Here's how the part is built. I have some questions about the finished solid (model axes, mm). A direction names the side the tool comes from. Coordinates: 2 decimals unless noted, no trailing zeros. Order: outer loops, then holes, each group sorted by start corner. A loop starts at its lowest first (then second) coordinate and runs counter-clockwise, first axis right, second up. Notation, with made-up numbers: (-9, 43.5) - (8, 43.5) arc R17 cw to (8, 69.5) - close; hole circle Ø8 at (-25.5, 50). An arc over 180 degrees is marked (long way). Answer in a Markdown table with one row per item. Add a question column.
Item 1: Will these pins go through, and if not, where does the flat tip stop? pin 1 Ø1 at (y, z) = (-5.5, -0.5) entering from +X; pin 2 Ø1.6 at (x, z) = (3, -0.5) entering from -Y; pin 3 Ø1 at (y, z) = (-7, 0.5) entering from -X.
Item 2: If I drill on line 1 along X through (y, z) = (-5, 1.4); line 2 along Y through (x, z) = (-10.5, -0.35), over which ranges is the centre line in solid material (lowest first)? Write a range as from..to.
Item 3: I want a section at C-C (x = 5). Please give me the cut outline in (y, z), plus the area to 3 significant figures.
Item 4: I want a section at A-A (y = -6). Please give me the cut outline in (x, z).
Item 5: I want a section at B-B (z = 0). Please give me the cut outline in (x, y).
Item 6: On a 3-axis mill with a long thin cutter (end or side, diameter ignored), from which of +Z, -Z, +X, -X, +Y, -Y can I reach the whole of each face in a straight line? I mean faces 1 (the flat face through (-38.202, -6, 0)), 2 (the flat face through (0, -4.864, 0)), 3 (the flat face through (40, -4.864, 0)). Say none if no direction works.
```python
from build123d import *

# Parameters (mm, degrees)
BOSS_EXTRUDE1_DEPTH = 1.5875
BOSS_EXTRUDE2_DEPTH = 3.175


with BuildPart() as part:
    # Sketch1 → Boss-Extrude1 (new body, symmetric)
    with BuildSketch(Plane.XY):
        Polygon((-12.6492, -4.7625), (12.7, -4.7625), (12.7, -7.9375), (38.1508, -7.9375), (38.1508, -4.7625), (41.275, -4.7625), (41.275, 4.7625), (-41.275, 4.7625), (-41.275, -4.7625), (-38.1, -4.7625), (-38.1, -7.9375), (-12.6492, -7.9375), align=None)
    extrude(amount=BOSS_EXTRUDE1_DEPTH, both=True)

    # Sketch2 → Boss-Extrude2 (add)
    with BuildSketch(Plane.XY.offset(1.5875)):
        Polygon((38.2524, -4.8641), (41.3766, -4.8641), (41.3766, 4.8641), (-41.3766, 4.8641), (-41.3766, -4.8641), (-38.2016, -4.8641), (-38.2016, -8.0391), (-12.5476, -8.0391), (-12.5476, -4.8641), (12.5984, -4.8641), (12.5984, -8.0391), (38.2524, -8.0391), align=None)
    extrude(amount=-BOSS_EXTRUDE2_DEPTH)


solid = part.part
```
Values follow:
| question | item | result |
|---|---|---|
| 1 | pin 1 | stops at x = 38.25 |
| 1 | pin 2 | stops at y = -4.86 |
| 1 | pin 3 | stops at x = -38.2 |
| 2 | line 1 | x = -38.2..-12.55, 12.6..38.25 |
| 2 | line 2 | y = -4.86..4.86 |
| 3 | outline | (-4.86, -1.59) - (4.86, -1.59) - (4.86, 1.59) - (-4.86, 1.59) - close |
| 3 | area | 30.9 mm^2 |
| 4 | outline | (-38.2, -1.59) - (-12.55, -1.59) - (-12.55, 1.59) - (-38.2, 1.59) - close; (12.6, -1.59) - (38.25, -1.59) - (38.25, 1.59) - (12.6, 1.59) - close |
| 5 | outline | (-41.38, -4.86) - (-38.2, -4.86) - (-38.2, -8.04) - (-12.55, -8.04) - (-12.55, -4.86) - (12.6, -4.86) - (12.6, -8.04) - (38.25, -8.04) - (38.25, -4.86) - (41.38, -4.86) - (41.38, 4.86) - (-41.38, 4.86) - close |
| 6 | face 1 | +Z, -Z, -X, -Y |
| 6 | face 2 | +Z, -Z, -Y |
| 6 | face 3 | +Z, -Z, +X, -Y |
